For this review, take the finished solid that the model builds, in its own axes (mm). Coordinates: 2 decimals unless noted, no trailing zeros. Order: outer loops, then holes, each group sorted by start corner. A loop starts at its lowest first (then second) coordinate and runs counter-clockwise, first axis right, second up.
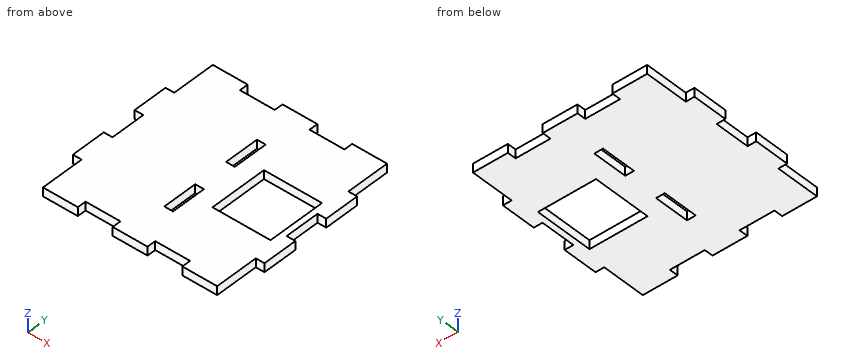
from build123d import *

# Parameters (mm, degrees)
ESBO_O1_W                = 3
ESBO_O1_H                = 12
ESBO_O1_W_2              = 20
ESBO_O1_H_2              = 20
RESSALTO_EXTRUS_O1_DEPTH = 3


with BuildPart() as part:
    # Esboço1 → Ressalto-extrusão1 (new body)
    with BuildSketch(Plane.XY):
        Polygon((-31.216896784, 10.517052385), (-31.216896784, -1.482947615), (-34.216896784, -1.482947615), (-34.216896784, -13.482947615), (-31.216896784, -13.482947615), (-31.216896784, -25.482947615), (-31.216896784, -28.482947615), (-19.216896784, -28.482947615), (-19.216896784, -25.482947615), (-7.216896784, -25.482947615), (-7.216896784, -28.482947615), (4.783103216, -28.482947615), (4.783103216, -25.482947615), (16.783103216, -25.482947615), (16.783103216, -28.482947615), (28.783103216, -28.482947615), (28.783103216, -25.482947615), (28.783103216, -13.482947615), (31.783103216, -13.482947615), (31.783103216, -1.482947615), (28.783103216, -1.482947615), (28.783103216, 10.517052385), (31.783103216, 10.517052385), (31.783103216, 22.517052385), (28.783103216, 22.517052385), (28.783103216, 34.517052385), (28.783103216, 37.517052385), (16.783103216, 37.517052385), (16.783103216, 34.517052385), (4.783103216, 34.517052385), (4.783103216, 37.517052385), (-7.216896784, 37.517052385), (-7.216896784, 34.517052385), (-19.216896784, 34.517052385), (-19.216896784, 37.517052385), (-31.216896784, 37.517052385), (-31.216896784, 34.517052385), (-31.216896784, 22.517052385), (-34.216896784, 22.517052385), (-34.216896784, 10.517052385), align=None)
        with Locations((-1.216896784, 16.517052385)):
            Rectangle(ESBO_O1_W, ESBO_O1_H, mode=Mode.SUBTRACT)
        with Locations((-1.216896784, -7.482947615)):
            Rectangle(ESBO_O1_W, ESBO_O1_H, mode=Mode.SUBTRACT)
        with Locations((16.783103216, 4.517052385)):
            Rectangle(ESBO_O1_W_2, ESBO_O1_H_2, mode=Mode.SUBTRACT)
    extrude(amount=RESSALTO_EXTRUS_O1_DEPTH)


solid = part.part
1. To check wall thickness, follow L1, parallel to X at y = -12, z = 0.75; L2, parallel to X at y = -4, z = 1.1; L3, parallel to Y at x = 18, z = 1.05. State the ranges of each line that lie inside material, in increasing order.
Answer below:
L1: x = -34.22 to -2.72, 0.28 to 31.78
L2: x = -34.22 to -2.72, 0.28 to 6.78, 26.78 to 31.78
L3: y = -28.48 to -5.48, 14.52 to 37.52
2. Take a section at A-A, the plane y = -10.5. Give the boundary of the cut face in (x, z), plus the area to 3 significant figures.
Answer below:
outline: (-34.22, 0) - (-2.72, 0) - (-2.72, 3) - (-34.22, 3) - close; (0.28, 0) - (31.78, 0) - (31.78, 3) - (0.28, 3) - close
area: 189 mm2
3. Take a section at C-C, the plane y = 12. Give the boundary of the cut face in (x, z), plus the area to 3 significant figures.
Answer below:
outline: (-34.22, 0) - (-2.72, 0) - (-2.72, 3) - (-34.22, 3) - close; (0.28, 0) - (6.78, 0) - (6.78, 3) - (0.28, 3) - close; (26.78, 0) - (31.78, 0) - (31.78, 3) - (26.78, 3) - close
area: 129 mm2
4. Clearance check with flat-ended pins moving along their axes: pin 1 Ø0.9 at (x, z) = (30.5, 1) entering from +Y; pin 2 Ø1.5 at (x, z) = (-32.5, 2) entering from -Y; pin 3 Ø1.5 at (y, z) = (28.5, 1.5) entering from +X. State where each tip first meets the part, or that it passes through.
Answer below:
pin 1: stops at y = 22.52
pin 2: stops at y = -13.48
pin 3: stops at x = 28.78
5. Take a section at D-D, the plane x = -15.5. Give the boundary of the cut face in (y, z).
Answer below:
outline: (-25.48, 0) - (34.52, 0) - (34.52, 3) - (-25.48, 3) - close
6. Take a section at B-B, the plane x = 21. Give the boundary of the cut face in (y, z), plus the area to 3 significant figures.
Answer below:
outline: (-28.48, 0) - (-5.48, 0) - (-5.48, 3) - (-28.48, 3) - close; (14.52, 0) - (37.52, 0) - (37.52, 3) - (14.52, 3) - close
area: 138 mm2
